Could you check a few things on this model? Use its own coordinates, in mm. Face numbers are marked on the shaded views. A direction names the side the tool comes from. Give positions to 0.01 mm unless a question says otherwise; leave off trailing zeros. Loops run counter-clockwise (first coordinate to the right, second up) from the corner with the lowest first, then second, coordinate; pieces in that order, holes last. Notation, with made-up numbers: (34, -26) - (45, -26) arc R16 ccw to (45, 2) - close; hole circle Ø4 at (44, 40.25). An arc over 180 degrees is marked (long way). One line per item, written item: value. Start each with the question number.
Q1. I'm going to push flat-ended pins straight in: P1, Ø1.5, axis at x = -7.5, y = 53, coming from the -Z side; P2, Ø8, axis at y = 41, z = -9, coming from the -X side; P3, Ø15.5, axis at x = 17.5, y = 45, coming from the +Z side; P4, Ø7, axis at x = -38, z = 0, coming from the -Y side. Where does each tip first touch, or does it pass through?
Q2. If I drill on line 1 (X direction, y = 28, z = 0); line 2 (Z direction, x = 38, y = 35); line 3 (X direction, y = 18, z = 0), over which ranges is the centre line in solid material (lowest first)? Write a range as from..to.
Q3. I want a section at A-A (z = 0). Please give me the cut outline in (x, y), then the cut area to 3 significant figures.
Q4. I want a section at B-B (y = 42). Please give me the cut outline in (x, z).
Q5. I want a section at C-C (z = 15.5). Please give me the cut outline in (x, y).
Q6. For the marked faces 4 and 5, which set-ups out of +Z, -Z, +X, -X, +Y, -Y let a thin tool reach every point of the face, with its end or its side?
Q7. If we mould it in two halves opening along Z, with no side actions, what happens to the marked faces 1, 2 and 3? For each: released by +Z, released by -Z, zero draft, split by the parting line, or undercut.
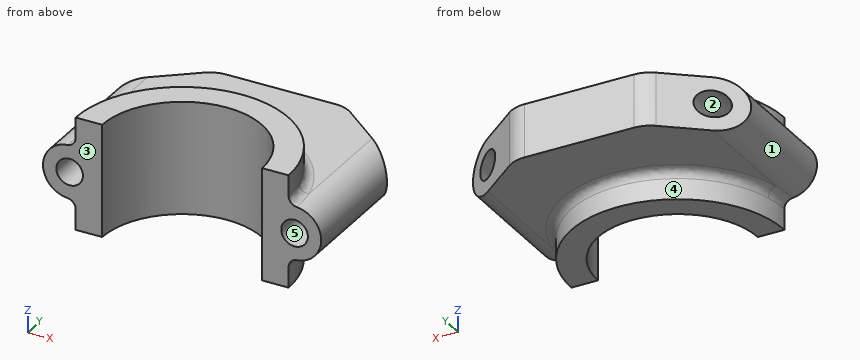
```python
from build123d import *

# Parameters (mm, degrees)
BOSS_EXTRUDE1_DEPTH     = 19
BOSS_EXTRUDE2_DEPTH     = 60
CUT_EXTRUDE1_DEPTH      = 29
SKETCH4_R               = 4.5
CUT_EXTRUDE2_DEPTH      = 61
CUT_EXTRUDE4_DEPTH      = 20
CUT_EXTRUDE4_DEPTH_BACK = 20
FILLET1_R               = 10
FILLET2_R               = 3


with BuildPart() as part:
    # Sketch1 → Boss-Extrude1 (new body, symmetric)
    with BuildSketch(Plane.XY):
        with BuildLine():
            Line((-36, 0), (-27, 0))
            ThreePointArc((-27, 0), (0, 27), (27, 0))
            Line((27, 0), (36, 0))
            ThreePointArc((36, 0), (0, 36), (-36, 0))
        make_face()
    extrude(amount=BOSS_EXTRUDE1_DEPTH, both=True)

    # Sketch2 → Boss-Extrude2 (add)
    with BuildSketch(Plane(origin=(0, 60, 0), x_dir=(-1, 0, 0), z_dir=(0, -1, 0))):
        with BuildLine():
            Line((38, -9), (-38, -9))
            ThreePointArc((-38, -9), (-47, 0), (-38, 9))
            Line((-38, 9), (38, 9))
            ThreePointArc((38, 9), (47, 0), (38, -9))
        make_face()
    extrude(amount=BOSS_EXTRUDE2_DEPTH)

    # Sketch3 → Cut-Extrude1 (cut, through all)
    with BuildSketch(Plane.XY.offset(9)):
        with BuildLine():
            Line((-27, 0), (27, 0))
            ThreePointArc((27, 0), (0, 27), (-27, 0))
        make_face()
    extrude(amount=-CUT_EXTRUDE1_DEPTH, mode=Mode.SUBTRACT)

    # Sketch4 → Cut-Extrude2 (cut, through all)
    with BuildSketch(Plane.XZ):
        with Locations((-38, 0)):
            Circle(SKETCH4_R)
        with Locations((38, 0)):
            Circle(SKETCH4_R)
    extrude(amount=-CUT_EXTRUDE2_DEPTH, mode=Mode.SUBTRACT)

    # Sketch5 → Cut-Extrude4 (cut, two sides)
    with BuildSketch(Plane.XY) as cut_extrude4_sk:
        Polygon((-47, 40), (-22, 60), (-47, 60), align=None)
        Polygon((47, 60), (47, 40), (22, 60), align=None)
    extrude(amount=CUT_EXTRUDE4_DEPTH, mode=Mode.SUBTRACT)
    extrude(cut_extrude4_sk.sketch, amount=-CUT_EXTRUDE4_DEPTH_BACK, mode=Mode.SUBTRACT)

    # Fillet1
    fillet1_edges = [part.edges().sort_by_distance(p)[0] for p in [
        (-22, 60, 0),
        (22, 60, 0),
    ]]
    fillet(fillet1_edges, radius=FILLET1_R)

    # Fillet2
    fillet2_edges = [part.edges().sort_by_distance(p)[0] for p in [
        (0, 36, 9),
        (0, 36, -9),
    ]]
    fillet(fillet2_edges, radius=FILLET2_R)


solid = part.part
```
Worked answers:
1. P1: stops at z = -9
1. P2: stops at x = -45.48
1. P3: stops at z = 9
1. P4: passes through
2. line 1: x = -47..-42.5, -33.5..33.5, 42.5..47
2. line 2: z = -9..-4.5, 4.5..9
2. line 3: x = -47..-42.5, -33.5..-20.12, 20.12..33.5, 42.5..47
3. outline: (-47, 0) - (-42.5, 0) - (-42.5, 43.6) - (-47, 40) - close; (-33.5, 0) - (-27, 0) arc R27 cw to (27, 0) - (33.5, 0) - (33.5, 50.8) - (24.74, 57.81) arc R10 ccw to (18.49, 60) - (-18.49, 60) arc R10 ccw to (-24.74, 57.81) - (-33.5, 50.8) - close; (42.5, 0) - (47, 0) - (47, 40) - (42.5, 43.6) - close
3. area: 3,140 mm²
4. outline: (-44.5, -6.22) arc R9 ccw to (-38, -9) - (38, -9) arc R9 ccw to (44.5, -6.22) - (44.5, 6.22) arc R9 ccw to (38, 9) - (-38, 9) arc R9 ccw to (-44.5, 6.22) - close; hole circle Ø9 at (-38, 0); hole circle Ø9 at (38, 0)
5. outline: (-36, 0) - (-27, 0) arc R27 cw to (27, 0) - (36, 0) arc R36 ccw to start
6. face 4: -Z, +Y
6. face 5: +Y, -Y
7. face 1: split by the parting line
7. face 2: undercut
7. face 3: zero draft
